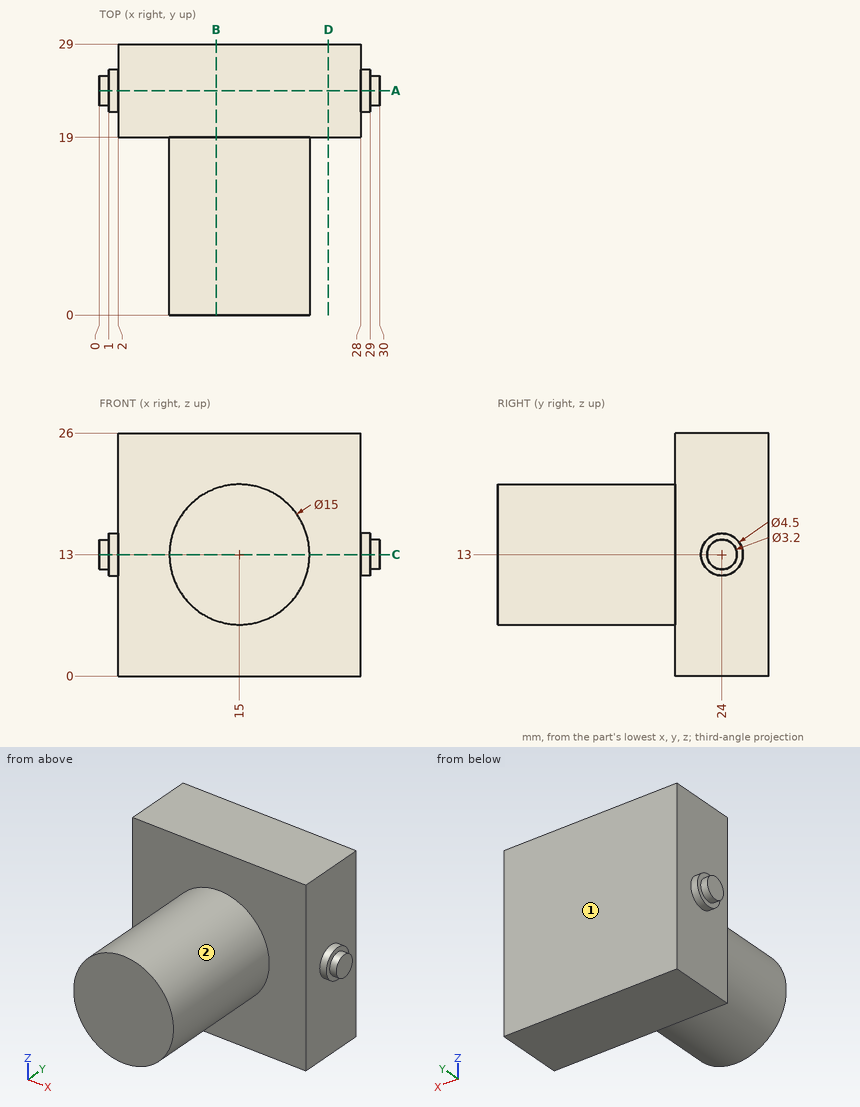
Job drawing, mm, ordinate dimensions from the low corner. One solid piece. A direction names the side the tool comes from. Coordinates: 2 decimals unless noted, no trailing zeros. Order: outer loops, then holes, each group sorted by start corner. A loop starts at its lowest first (then second) coordinate and runs counter-clockwise, first axis right, second up. Notation, with made-up numbers: (60.25, -13.5) -> (72.25, -13.5) arc R26 cw to (72.25, 13.5) -> close; hole circle Ø7 at (-10, -26). An arc over 180 degrees is marked (long way). Answer in a Markdown table with one row per item. Add a question column.
Q1. Band-saw the part on C-C, the plane z = 13. List the corners of the cut face in (x, y).
Q2. Drop flat-ended pins along their axis: pin 1 (3 mm diameter, centred on x = 21.5, y = 13, fed in from -Z); pin 2 (5 mm diameter, centred on y = 26.5, z = 18, fed in from -X); pin 3 (6 mm diameter, centred on x = 16.5, z = 21.5, fed in from -Y); pin 4 (3 mm diameter, centred on y = 7, z = 20, fed in from +X). Give the stop position or say it passes through.
Q3. Band-saw the part on D-D, the plane x = 24.5. List the corners of the cut face in (y, z), then the cut area to 3 significant figures.
Q4. Which spindle directions (+Z, -Z, +X, -X, +Y, -Y) get a long thin tool onto all of the face, cutting with end or side? Do the marked faces 1 and 2. Say none if no direction does.
Q5. Band-saw the part on B-B, the plane x = 12.5. List the corners of the cut face in (y, z).
Q6. Band-saw the part on A-A, the plane y = 24. List the corners of the cut face in (x, z).
Q7. Wall check: line 1 along Y through (x, z) = (21.5, 18.5); line 2 along X through (y, z) = (20, 12); line 3 along X through (y, z) = (8.5, 7.5). Give the ranges that are in metal, low to high. Write a range as [from, to].
Answers follow:
| question | item | result |
|---|---|---|
| 1 | outline | (0, 22.4) -> (1, 22.4) -> (1, 21.75) -> (2, 21.75) -> (2, 19) -> (7.5, 19) -> (7.5, 0) -> (22.5, 0) -> (22.5, 19) -> (28, 19) -> (28, 21.75) -> (29, 21.75) -> (29, 22.4) -> (30, 22.4) -> (30, 25.6) -> (29, 25.6) -> (29, 26.25) -> (28, 26.25) -> (28, 29) -> (2, 29) -> (2, 26.25) -> (1, 26.25) -> (1, 25.6) -> (0, 25.6) -> close |
| 2 | pin 1 | z = 7.41 |
| 2 | pin 2 | x = 2 |
| 2 | pin 3 | y = 0 |
| 2 | pin 4 | x = 20.1 |
| 3 | outline | (19, 0) -> (29, 0) -> (29, 26) -> (19, 26) -> close |
| 3 | area | 260 mm^2 |
| 4 | face 1 | +Z, -Z, +X, -X, +Y |
| 4 | face 2 | -Y |
| 5 | outline | (0, 5.93) -> (19, 5.93) -> (19, 0) -> (29, 0) -> (29, 26) -> (19, 26) -> (19, 20.07) -> (0, 20.07) -> close |
| 6 | outline | (0, 11.4) -> (1, 11.4) -> (1, 10.75) -> (2, 10.75) -> (2, 0) -> (28, 0) -> (28, 10.75) -> (29, 10.75) -> (29, 11.4) -> (30, 11.4) -> (30, 14.6) -> (29, 14.6) -> (29, 15.25) -> (28, 15.25) -> (28, 26) -> (2, 26) -> (2, 15.25) -> (1, 15.25) -> (1, 14.6) -> (0, 14.6) -> close |
| 7 | line 1 | [19, 29] |
| 7 | line 2 | [2, 28] |
| 7 | line 3 | [9.9, 20.1] |
